Could you check a few things on this drawing? It's one solid part, dimensions in mm from its lowest x, y, z. A direction names the side the tool comes from. Coordinates: 2 decimals unless noted, no trailing zeros. Loops run counter-clockwise (first coordinate to the right, second up) from the corner with the lowest first, then second, coordinate; pieces in that order, holes last.
1) If I drill on line 1 along Z through (x, y) = (360.5, 106); line 2 along Y through (x, z) = (111, 203.5); line 3 along Z through (x, y) = (311, 42), over which ranges is the centre line in solid material (lowest first)?
2) Imagine slicing it at A-A on x = 325. Please give me the cut outline in (y, z), plus the area to 3 significant figures.
3) Imagine slicing it at D-D on x = 149. Please give me the cut outline in (y, z), plus the area to 3 significant figures.
4) Will these pins go through, and if not, where does the flat tip stop? P1, Ø4, axis at x = 163, y = 115, coming from the -Z side; P2, Ø2, axis at x = 328.5, z = 133.5, coming from the +Y side; P3, Ø7.5, axis at y = 107.5, z = 41, coming from the -X side (3 decimals).
5) Imagine slicing it at C-C on z = 211. Please give me the cut outline in (x, y), plus the area to 3 significant figures.
6) For the marked faces 1, 2 and 3, which set-ups out of +Z, -Z, +X, -X, +Y, -Y let a thin tool reach every point of the face, with its end or its side?
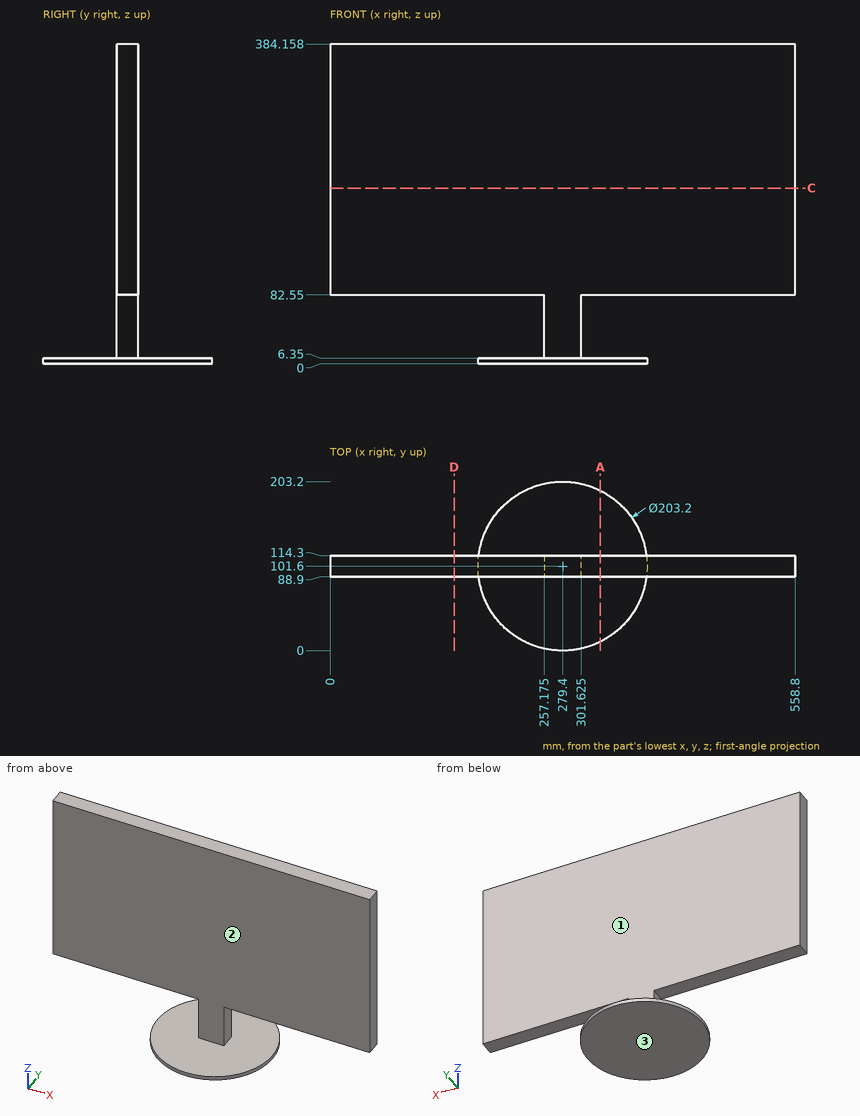
Filled in:
1. line 1: z = 0 to 6.35, 82.55 to 384.16
1. line 2: y = 88.9 to 114.3
1. line 3: z = 0 to 6.35
2. outline: (10.81, 0) - (192.39, 0) - (192.39, 6.35) - (10.81, 6.35) - close; (88.9, 82.55) - (114.3, 82.55) - (114.3, 384.16) - (88.9, 384.16) - close
2. area: 8,810 mm2
3. outline: (88.9, 82.55) - (114.3, 82.55) - (114.3, 384.16) - (88.9, 384.16) - close
3. area: 7,660 mm2
4. P1: stops at z = 82.55
4. P2: stops at y = 114.3
4. P3: stops at x = 257.175
5. outline: (0, 88.9) - (558.8, 88.9) - (558.8, 114.3) - (0, 114.3) - close
5. area: 14,200 mm2
6. face 1: +Z, +X, -X, +Y
6. face 2: +Z, +X, -X, -Y
6. face 3: -Z, +X, -X, +Y, -Y
